```python
from build123d import *

# Parameters (mm, degrees)
F1_DEPTH    = 18
F2_T1_DEPTH = 18
F2_T3_DEPTH = 46.2017417965
F3_R        = 22.3056916506
F4_R        = 15.8040911287
F5_R        = 1.7635852265
F5_R_2      = 3.1709752344
F6_DEPTH    = 18


# Not quite as in the source:
# - a fillet or chamfer that OpenCascade refuses, or shapes differently, is made with other operations: its cross-section is extruded or revolved along the edge and cut away or added


with BuildPart() as f1:
    # F0 (on Top) → F1 (new body)
    with BuildSketch(Plane.XY):
        Polygon((-17.5491029148, 7.6061424899), (7.4508970852, 7.6061424899), (7.4508970852, -54.8938575101), (11.4508970852, -48.259973526), (11.4508970852, 24.6061424899), (7.4508970852, 24.6061424899), (-5.5491029148, 12.6061424899), (-17.5491029148, 12.6061424899), (-29.5491029148, 4.6061424899), (-17.5491029148, 4.6061424899), align=None)
    extrude(amount=F1_DEPTH)

    # F2: fillet of radius 14.9219158343 on 2 edges, made by hand

    # F2_s2 → F2_t1 (join)
    with BuildSketch(Plane.XY):
        with BuildLine():
            ThreePointArc((-11.3833307845, 12.6061424899), (-5.9496574254, 13.6306209347), (-1.2620921794, 16.5633831687))
            Line((-1.2620921794, 16.5633831687), (-5.5491029148, 12.6061424899))
            Line((-5.5491029148, 12.6061424899), (-11.3833307845, 12.6061424899))
        make_face()
    extrude(amount=F2_T1_DEPTH)

    # F2_s4 → F2_t3 (cut)
    with BuildSketch(Plane.XY.offset(-14.1008708982)):
        with BuildLine():
            ThreePointArc((11.4508970852, 24.6061424899), (7.0833751355, 23.32182366), (3.3063496819, 20.7804064253))
            Line((3.3063496819, 20.7804064253), (7.4508970852, 24.6061424899))
            Line((7.4508970852, 24.6061424899), (11.4508970852, 24.6061424899))
        make_face()
    extrude(amount=F2_T3_DEPTH, mode=Mode.SUBTRACT)

    # F3
    f3_edges = [f1.edges().sort_by_distance(p)[0] for p in [
        (-17.549103, 12.606142, 9),
    ]]
    fillet(f3_edges, radius=F3_R)

    # F4
    f4_edges = [f1.edges().sort_by_distance(p)[0] for p in [
        (11.450897, -48.259974, 9),
    ]]
    fillet(f4_edges, radius=F4_R)

    # F5 (on face) → F6 (cut)
    with BuildSketch(Plane.XY.offset(18)):
        with Locations((-1.5691251028, 11.2882275134)):
            Circle(F5_R)
        with Locations((5.2787014283, 13.1632275879)):
            Circle(F5_R_2)
        with Locations((7.8058750369, 19.5219237357)):
            Circle(F5_R)
    extrude(amount=-F6_DEPTH, mode=Mode.SUBTRACT)


solid = f1.part
```
The listing builds one solid part. Answer for the finished solid, in the listing's coordinates (mm). A direction names the side the tool comes from. Round coordinates to 2 decimals unless told otherwise and drop trailing zeros. Loops run counter-clockwise (first coordinate to the right, second up) from the corner with the lowest first, then second, coordinate; pieces in that order, holes last. Notation, with made-up numbers: (88, 59) - (99, 59) arc R17 ccw to (99, 83) - close; hole circle Ø7 at (66, 33). An arc over 180 degrees is marked (long way). Use one line per item in the form item = value. Start each with the question number.
1. Consider line 1 (Y direction, x = 6.5, z = 2.75); line 2 (X direction, y = -26, z = 10.5); line 3 (Y direction, x = -11, z = 15). Determine where each line is inside the solid, lowest interval first. Write a range as [from, to].
2. The part is cut by section C-C on y = -47.5. Determine the outline of the cut face in (x, z), then the cut area to 3 significant figures.
3. For a pull along X with two mould halves and no side action, classify faces 3 (the face through (-5.91, 13.646, 8.874)), 4 (the face through (-5, 7.606, 9)), 5 (the face through (8, -3, 0)), 6 (the face through (-17.549, 6, 9)) as pulls with the +X half, pulls with the -X half, needs draft (parallel to the pull), parting line crosses it, or undercut.
4. The part is cut by section B-B on y = 3. Determine the outline of the cut face in (x, z), then the cut area to 3 significant figures.
5. The part is cut by section A-A on z = 7.5. Give the number of separate pieces and of enclosed holes in the cut face, then the cut area to 3 significant figures.
6. Given pin 1 Ø5.5 at (x, z) = (-11, 7.5) entering from -Y; pin 2 Ø5.5 at (y, z) = (-27.5, 5) entering from -X; pin 3 Ø10 at (x, z) = (-23.5, 6) entering from -Y, each flat-ended and moving along its own axis, determine where each tip first touches the part or whether it passes through.
7. A tool of negligible diameter and unlimited length cuts with its end or side. For faces 1 (the face through (-24, 4.606, 9)), 2 (the face through (10.9, -48, 9.1)), from which of +Z, -Z, +X, -X, +Y, -Y can it reach the whole face along a straight path? Write none if from no direction.
Geometry check:
q1.line_1 = [7.61, 10.24], [16.09, 18.34], [20.71, 23.03]
q1.line_2 = [7.45, 11.45]
q1.line_3 = [7.61, 12.61]
q2.outline = (7.45, 0) - (11.03, 0) - (11.03, 18) - (7.45, 18) - close
q2.area = 64.4 mm^2
q3.face_3 = pulls with the -X half
q3.face_4 = undercut
q3.face_5 = needs draft
q3.face_6 = undercut
q4.outline = (7.45, 0) - (11.45, 0) - (11.45, 18) - (7.45, 18) - close
q4.area = 72.0 mm^2
q5.separate_pieces = 1
q5.enclosed_holes = 3
q5.area = 499 mm^2
q6.pin_1 = 7.61
q6.pin_2 = 7.45
q6.pin_3 = 4.61
q7.face_1 = +Z, -Z, -X, -Y
q7.face_2 = +Z, -Z, +X, -Y
